Verification items for the finished model (mm, model axes). A direction names the side the tool comes from. Round coordinates to 2 decimals unless told otherwise and drop trailing zeros. Order: outer loops, then holes, each group sorted by start corner. A loop starts at its lowest first (then second) coordinate and runs counter-clockwise, first axis right, second up. Notation, with made-up numbers: (32.5, 46) -> (70.5, 46) arc R23 cw to (70.5, 83) -> close; hole circle Ø11 at (-20.75, 63.5). An arc over 180 degrees is marked (long way). Return JSON: item names as keys, results as strings. Group by question number.
1) Section check A-A on z = 62.75. Enter the section's corners in (x, y), plus the area to 3 significant figures.
2) Draft check along Y on faces 1 (the flat face through (20.685, 129.008, 63.972)), 2 (the cylindrical face through (19.38, 124.94, 64.03)), 3 (the cylindrical face through (39.3, 121.4, 65)). Enter one of: pulls with the +Y half, pulls with the -Y half, needs draft (parallel to the pull), parting line crosses it, or undercut.
3) Scan lines: L1, parallel to Z at x = 27, y = 130.25; L2, parallel to Y at x = 35.75, z = 67.5; L3, parallel to X at y = 118.5, z = 68. Record each from-to range of solid material in increasing order.
4) Depth check by flat-ended pin: pin 1 (1.5 mm diameter, centred on x = 34, z = 66, fed in from -Y); pin 2 (3 mm diameter, centred on x = 39, y = 119, fed in from +Z); pin 3 (1.5 mm diameter, centred on x = 29, y = 122, fed in from +Z). Enter the tip coordinate at first touch or a pass-through.
5) Section check B-B on x = 24.25. Enter the section's corners in (y, z).
6) Section check D-D on z = 69.5. Enter the section's corners in (x, y), plus the area to 3 significant figures.
7) Tool access check on faces 4 (the flat face through (37, 116, 71)), 5 (the flat face through (38, 119, 64)). Record the directions out of +Z, -Z, +X, -X, +Y, -Y that give a thin tool (end or side, any length) a straight path to the whole face; none if there is none.
```python
from build123d import *

# Parameters (mm, degrees)
CYLINDER081_R          = 2.75
CYLINDER081_DEPTH      = 7
CYLINDER078_R          = 4
CYLINDER078_DEPTH      = 9
CYLINDER071_R          = 1.38
CYLINDER071_DEPTH      = 10
CYLINDER069_R          = 2.75
CYLINDER069_DEPTH      = 10
BOX039_W               = 25
BOX039_H               = 10
BOX039_DEPTH           = 4
CUT049_PLACEMENT_ANGLE = 30
FILLET006_R            = 3


with BuildPart() as cilindro002:
    # Cylinder081 → Cylinder081 (new body)
    with BuildSketch(Plane(origin=(17, 17, 12), x_dir=(1, 0, 0), z_dir=(0, 0, 1))):
        Circle(CYLINDER081_R)
    extrude(amount=CYLINDER081_DEPTH)


with BuildPart() as obj1:
    # Cylinder078 → Cylinder078 (new body)
    with BuildSketch(Plane(origin=(17, 17, 10), x_dir=(1, 0, 0), z_dir=(0, 0, 1))):
        Circle(CYLINDER078_R)
    extrude(amount=CYLINDER078_DEPTH)

    # Cut053: cut Cilindro002
    add(cilindro002.part, mode=Mode.SUBTRACT)


with BuildPart() as obj1_1:
    # Cut053 placement: moved
    add(obj1.part.moved(Location((21, 102, 52))))


with BuildPart() as cylinder071:
    # Cylinder071 → Cylinder071 (new body)
    with BuildSketch(Plane(origin=(25, 52, 59), x_dir=(1, 0, 0), z_dir=(0, 0, 1))):
        Circle(CYLINDER071_R)
    extrude(amount=CYLINDER071_DEPTH)


with BuildPart() as cylinder069:
    # Cylinder069 → Cylinder069 (new body)
    with BuildSketch(Plane(origin=(40, 52, 59), x_dir=(1, 0, 0), z_dir=(0, 0, 1))):
        Circle(CYLINDER069_R)
    extrude(amount=CYLINDER069_DEPTH)


with BuildPart() as fusion009:
    # Box039 → Box039 (new body)
    with BuildSketch(Plane(origin=(45, 57, 62), x_dir=(-1, 0, 0), z_dir=(0, 0, 1))):
        with Locations((12.5, 5)):
            Rectangle(BOX039_W, BOX039_H)
    extrude(amount=BOX039_DEPTH)

    # Cut046: cut Cylinder069
    add(cylinder069.part, mode=Mode.SUBTRACT)

    # Cut049: cut Cylinder071
    add(cylinder071.part, mode=Mode.SUBTRACT)


with BuildPart() as fusion009_1:
    # Cut049 placement: moved
    add(fusion009.part.moved(Location((-20.65, 26.95, 0))).rotate(Axis((-20.65, 26.95, 0), (0, 0, -1)), CUT049_PLACEMENT_ANGLE))

    # Fillet006
    fillet006_edges = [fusion009_1.edges().sort_by_distance(p)[0] for p in [
        (25.170508, 66.313448, 64),
        (20.170508, 57.653194, 64),
    ]]
    fillet(fillet006_edges, radius=FILLET006_R)


with BuildPart() as fusion009_2:
    # Fillet006 placement: moved
    add(fusion009_1.part.moved(Location((-2, 67, 0))))

    # Fusion009: union obj1
    add(obj1_1.part)


solid = fusion009_2.part
```
Check result:
{
 "1": {"outline": "(19.67, 127.25) arc R3 ccw to (20.77, 123.15) -> (39.82, 112.15) -> (44.82, 120.81) -> (25.77, 131.81) arc R3 ccw to (21.67, 130.72) -> close; hole circle Ø2.76 at (25, 126.48)", "area": "240 mm^2"},
 "2": {"face 1": "pulls with the +Y half", "face 2": "parting line crosses it", "face 3": "undercut"},
 "3": {"L1": "62 to 66", "L2": "115.69 to 117.42, 120.58 to 122.31", "L3": "34.03 to 35.3, 40.7 to 41.97"},
 "4": {"pin 1": "y = 115.08", "pin 2": "z = 64", "pin 3": "z = 66"},
 "5": {"outline": "(121.14, 62) -> (125.33, 62) -> (125.33, 66) -> (121.14, 66) -> close; (127.64, 62) -> (132.22, 62) -> (132.22, 66) -> (127.64, 66) -> close"},
 "6": {"outline": "circle Ø8 at (38, 119); hole circle Ø5.5 at (38, 119)", "area": "26.5 mm^2"},
 "7": {"face 4": "+Z, +X, -X, +Y, -Y", "face 5": "+Z"}
}
